Design review of the part built by this model. Coordinates are the model's own, in mm. Face numbers are marked on the shaded views. Round coordinates to 2 decimals unless told otherwise and drop trailing zeros. Write each loop counter-clockwise with the first axis right and the second up, starting at its lowest first coordinate (ties: lowest second). Pieces come first, ordered by that corner, then holes. Notation, with made-up numbers: M -14,65 L 23,65 A21 cw 23,100 Z; hole C 72.5,-6 d9. An arc over 180 degrees is marked long. One line per question, with ' | ' between items. Start each with the question number.
Item 1: Add section A-A, the plane y = -54.5. State the section outline as (x, z) points, and give its area (3 significant figures).
Item 2: Add section C-C, the plane z = 132. State the section outline as (x, y) points, and give its area (3 significant figures).
Item 3: Draft analysis for pull direction Y (two halves, no side actions). For the marked faces 1 and 2, state which applies: released by +Y, released by -Y, zero draft, split by the parting line, or undercut.
Item 4: Insertion check: pin 1 Ø10 at (x, z) = (35, 86.5) entering from +Y; pin 2 Ø3.5 at (x, z) = (0, -164.58) entering from -Y; pin 3 Ø10 at (x, z) = (57, 118) entering from +Y. Each pin has a flat end and moves straight along its axis. Give the tip position at first contact, or say it passes through.
Item 5: For L1, parallel to Z at x = 0, y = 71.5; L2, parallel to Y at x = 0, z = 62; L3, parallel to X at y = -9, z = -192, list the stretches that pass through material, from the lowest coordinate up.
Item 6: Add section B-B, the plane x = -39. State the section outline as (y, z) points, and give its area (3 significant figures).
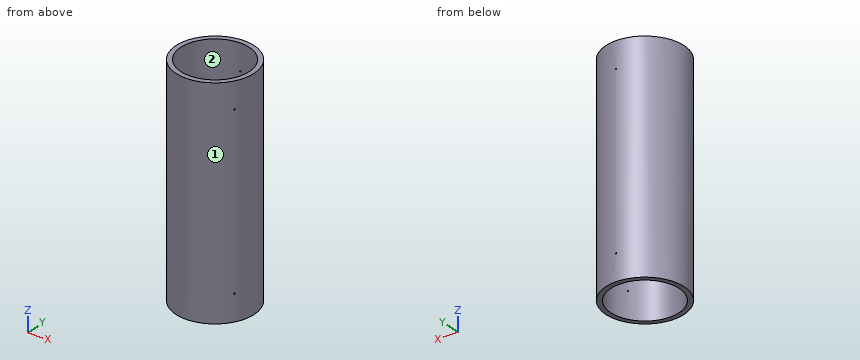
```python
from build123d import *

# Parameters (mm, degrees)
SKETCH1_R                  = 76.1746
SKETCH1_R_2                = 66.6496
BOSS_EXTRUDE1_DEPTH        = 215.3793
F_4_40_TAPPED_HOLE1_REACH  = 418.391
F_4_40_TAPPED_HOLE1_BORE_R = 1.1303
CIRPATTERN1_COUNT          = 3
MIRROR1_COPY_1_REACH       = 418.391
MIRROR1_COPY_1_SKETCH_R    = 1.1303
MIRROR1_COPY_2_REACH       = 418.391
MIRROR1_COPY_2_SKETCH_R    = 1.1303


with BuildPart() as part:
    # Sketch1 → Boss-Extrude1 (new, symmetric)
    with BuildSketch(Plane.XY):
        Circle(SKETCH1_R)
        Circle(SKETCH1_R_2, mode=Mode.SUBTRACT)
    extrude(amount=BOSS_EXTRUDE1_DEPTH, both=True)

    # #4-40 Tapped Hole1 bore (on position points) → #4-40 Tapped Hole1 (cut, up to next)
    with BuildSketch(Plane(origin=(0, 76.1746, 164.5793), x_dir=(1, 0, 0), z_dir=(0, 1, 0)), mode=Mode.PRIVATE) as f_4_40_tapped_hole1_sk1:
        Circle(F_4_40_TAPPED_HOLE1_BORE_R)
    f_4_40_tapped_hole1_tool1 = extrude(f_4_40_tapped_hole1_sk1.sketch, amount=-F_4_40_TAPPED_HOLE1_REACH, mode=Mode.PRIVATE) & part.part
    f_4_40_tapped_hole1 = f_4_40_tapped_hole1_tool1.solids().sort_by_distance((0, 76.1746, 164.5793))[0]
    add(f_4_40_tapped_hole1, mode=Mode.SUBTRACT)

    # CirPattern1: #4-40 Tapped Hole1 ×3 about axis
    cirpattern1_axis = Axis((0, 0, 215.3793), (0, 0, 1))
    for i in range(1, CIRPATTERN1_COUNT):
        add(f_4_40_tapped_hole1.rotate(cirpattern1_axis, i * 360 / CIRPATTERN1_COUNT), mode=Mode.SUBTRACT)

    # Mirror1: #4-40 Tapped Hole1 across plane
    add(f_4_40_tapped_hole1.mirror(Plane.XY), mode=Mode.SUBTRACT)

    # Mirror1 copy 1 sketch → Mirror1 copy 1 (cut, up to next)
    with BuildSketch(Plane(origin=(-65.969138723, -38.0873, -164.5793), x_dir=(-0.4999999999999998, 0.8660254037844387, 0), z_dir=(-0.8660254037844387, -0.4999999999999998, 0)), mode=Mode.PRIVATE) as mirror1_copy_1_sk1:
        Circle(MIRROR1_COPY_1_SKETCH_R)
    mirror1_copy_1_tool1 = extrude(mirror1_copy_1_sk1.sketch, amount=-MIRROR1_COPY_1_REACH, mode=Mode.PRIVATE) & part.part
    add(mirror1_copy_1_tool1.solids().sort_by_distance((-65.969138723, -38.0873, -164.5793))[0], mode=Mode.SUBTRACT)

    # Mirror1 copy 2 sketch → Mirror1 copy 2 (cut, up to next)
    with BuildSketch(Plane(origin=(65.969138723, -38.0873, -164.5793), x_dir=(-0.5000000000000004, -0.8660254037844384, 0), z_dir=(0.8660254037844384, -0.5000000000000004, 0)), mode=Mode.PRIVATE) as mirror1_copy_2_sk1:
        Circle(MIRROR1_COPY_2_SKETCH_R)
    mirror1_copy_2_tool1 = extrude(mirror1_copy_2_sk1.sketch, amount=-MIRROR1_COPY_2_REACH, mode=Mode.PRIVATE) & part.part
    add(mirror1_copy_2_tool1.solids().sort_by_distance((65.969138723, -38.0873, -164.5793))[0], mode=Mode.SUBTRACT)


solid = part.part
```
Computed values:
1) outline: M -53.22,-215.38 L -38.37,-215.38 L -38.37,215.38 L -53.22,215.38 Z; M 38.37,-215.38 L 53.22,-215.38 L 53.22,215.38 L 38.37,215.38 Z | area: 12,800 mm^2
2) outline: C 0,0 d152.35; hole C 0,0 d133.3 | area: 4,270 mm^2
3) face 1: split by the parting line | face 2: undercut
4) pin 1: stops at y = 70.02 | pin 2: stops at y = -76.17 | pin 3: stops at y = 55.66
5) L1: z = -215.38 to -165.71, -163.45 to 163.45, 165.71 to 215.38 | L2: y = -76.17 to -66.65, 66.65 to 76.17 | L3: x = -75.64 to -66.04, 66.04 to 75.64
6) outline: M -65.43,-215.38 L -54.05,-215.38 L -54.05,215.38 L -65.43,215.38 Z; M 54.05,-215.38 L 65.43,-215.38 L 65.43,215.38 L 54.05,215.38 Z | area: 9,810 mm^2
